The listing builds one solid part. Answer for the finished solid, in the listing's coordinates (mm). A direction names the side the tool comes from. Give positions to 0.01 mm unless a question says otherwise; leave off trailing zeros. Write each loop counter-clockwise with the first axis right and the second up, starting at its lowest first coordinate (ties: lowest second). Pieces come first, ordered by that corner, then holes. Notation, with made-up numbers: (78, 78) -> (131, 78) arc R13 ccw to (131, 82) -> close; hole circle Ø11 at (62, 85). An arc over 180 degrees is marked (long way). Use CSV: the item, a comma, the result in double quotes. Start each with the question number.
from build123d import *

# Parameters (mm, degrees)
BOSS_EXTRUDE1_DEPTH     = 6.35
CUT_EXTRUDE1_START      = -9.525
SKETCH2_R               = 2.286
SKETCH2_R_2             = 2.285999999999999
CUT_EXTRUDE1_DEPTH      = 19.05
CUT_EXTRUDE2_DEPTH      = 15.892070207999966
CUT_EXTRUDE2_DEPTH_BACK = 15.892070207999966
SKETCH3_R               = 2.286
BOSS_EXTRUDE2_DEPTH     = 3.048
BOSS_EXTRUDE3_REACH     = 17.642
FILLET1_R               = 2.54
FILLET2_R               = 0.762


with BuildPart() as part:
    # Sketch1 → Boss-Extrude1 (new body)
    with BuildSketch(Plane(origin=(0, 0, 0), x_dir=(1, 0, 0), z_dir=(0, 1, 0))):
        with BuildLine():
            Line((6.984999999999984, -9.525000000000002), (-6.98499999999998, -9.525000000000006))
            ThreePointArc((-6.98499999999998, -9.525000000000006), (-8.78105122421383, -8.781051224213837), (-9.524999999999999, -6.984999999999987))
            Line((-9.524999999999999, -6.984999999999987), (-9.524999999999999, 6.984999999999979))
            ThreePointArc((-9.524999999999999, 6.984999999999979), (-8.78105122421383, 8.781051224213828), (-6.984999999999981, 9.524999999999997))
            Line((-6.984999999999981, 9.524999999999997), (6.984999999999984, 9.525))
            ThreePointArc((6.984999999999984, 9.525), (8.781051224213833, 8.781051224213831), (9.525000000000002, 6.984999999999983))
            Line((9.525000000000002, 6.984999999999983), (9.525000000000002, -6.984999999999984))
            ThreePointArc((9.525000000000002, -6.984999999999984), (8.781051224213833, -8.781051224213833), (6.984999999999984, -9.525000000000002))
        make_face()
    extrude(amount=BOSS_EXTRUDE1_DEPTH)

    # Sketch2 → Cut-Extrude1 (cut)
    with BuildSketch(Plane.XY.offset(CUT_EXTRUDE1_START)):
        with Locations(Location((-4.7624999999999975, 3.175, 0), (0, 0, 166.463797263))):
            Circle(SKETCH2_R)
        with Locations(Location((4.762500000000003, 3.175, 0), (0, 0, 13.536202737))):
            Circle(SKETCH2_R_2)
    extrude(amount=CUT_EXTRUDE1_DEPTH, mode=Mode.SUBTRACT)

    # Sketch3 → Cut-Extrude2 (cut, two sides: drawn at the far end of the back side and taken through both)
    with BuildSketch(Plane(origin=(0, 0, 0), x_dir=(0, 0, -1), z_dir=(1, 0, 0)).offset(-CUT_EXTRUDE2_DEPTH_BACK)):
        with Locations(Location((-4.7625, 3.175, 0), (0, 0, 90))):
            Circle(SKETCH3_R)
        with Locations(Location((4.7625, 3.175, 0), (0, 0, 90))):
            Circle(SKETCH3_R)
    extrude(amount=CUT_EXTRUDE2_DEPTH + CUT_EXTRUDE2_DEPTH_BACK, mode=Mode.SUBTRACT)


with BuildPart() as body_2:
    # Sketch4 → Boss-Extrude2 (new, symmetric)
    with BuildSketch(Plane.XY):
        Polygon((-6.35, -3.175), (6.35, -3.1749999999999985), (6.350000000000001, -4.775199999999996), (3.175, -7.950199999999998), (-3.174999999999998, -7.950199999999998), (-6.35, -4.775199999999998), align=None)
    extrude(amount=BOSS_EXTRUDE2_DEPTH, both=True)

    # Sketch5 → Boss-Extrude3 (add, up to next)
    with BuildSketch(Plane.XZ, mode=Mode.PRIVATE) as boss_extrude3_sk1:
        with BuildLine():
            Line((3.0479999999999996, -3.0479999999999996), (0, -3.048))
            ThreePointArc((0, -3.048), (-2.155261469056597, -2.155261469056597), (-3.0479999999999996, 4.3e-16))
            Line((-3.0479999999999996, 4.3e-16), (-3.048000000000001, 3.048))
            Line((-3.048000000000001, 3.048), (0, 3.048))
            ThreePointArc((0, 3.048), (2.1552614690565965, 2.155261469056597), (3.0479999999999996, 4.3e-16))
            Line((3.0479999999999996, 4.3e-16), (3.0479999999999996, -3.0479999999999996))
        make_face()
    boss_extrude3_tool1 = extrude(boss_extrude3_sk1.sketch, amount=BOSS_EXTRUDE3_REACH, mode=Mode.PRIVATE) - body_2.part

    add(part.part)  # Boss-Extrude3 merges part
    add(boss_extrude3_tool1.solids().sort_by_distance((0, 0, 0))[0])

    # Sketch6 → Revolve1 (revolve)
    with BuildSketch(Plane.XY):
        with BuildLine():
            Line((-6.349999999999999, -1.016), (-6.349999999999999, 0))
            Line((-6.349999999999999, 0), (-8.889999999999999, 0))
            ThreePointArc((-8.889999999999999, 0), (-7.717831861012163, -0.7525796525304105), (-6.349999999999999, -1.016))
        make_face()
    revolve1 = revolve(axis=Axis((-6.349999999999999, 0, 0), (0, 1, 0)))

    # Mirror1: Revolve1 across plane
    add(revolve1.mirror(Plane(origin=(0, 0, 0), x_dir=(0, 0, 1), z_dir=(1, 0, 0))))

    # Fillet1
    fillet1_edges = [body_2.edges().sort_by_distance(p)[0] for p in [
        (-6.35, -3.975099999999999, -3.048),
        (6.3500000000000005, -3.9750999999999976, 3.048),
    ]]
    fillet(fillet1_edges, radius=FILLET1_R)

    # Fillet2
    # the kernel refuses this fillet: 0.762 mm, written as the material it adds along each edge
    with BuildSketch(Plane(origin=(-6.349999999999999, 0, 0), x_dir=(-1, 0, 0), z_dir=(0, 0, -1))) as fillet2_piece_1:
        with BuildLine():
            CenterArc((2.8284242963176522, -0.762), FILLET2_R, 90, 39.51765279717284)
            ThreePointArc((2.3435515598060546, -0.17417142857142887), (2.443328238479981, -0.08883673664575209), (2.54, 0))
            Line((2.54, 0), (2.8284242963176522, 0))
        make_face()
    revolve(axis=Axis((-6.349999999999999, 0, 0), (0, 1, 0)))
    with BuildSketch(Plane(origin=(6.349999999999999, 0, 0), x_dir=(1, 0, 0), z_dir=(0, 0, -1))) as fillet2_piece_2:
        with BuildLine():
            CenterArc((2.8284242963176522, 0.762), FILLET2_R, 230.48234720282716, 39.51765279717284)
            ThreePointArc((2.3435515598060546, 0.17417142857142887), (2.443328238479981, 0.08883673664575209), (2.54, 0))
            Line((2.54, 0), (2.8284242963176522, 0))
        make_face()
    revolve(axis=Axis((6.349999999999999, 0, 0), (0, -1, 0)))
    # the kernel refuses this fillet: 0.762 mm, written as the material it takes off along each edge
    with BuildSketch(Plane(origin=(3.0479999999999996, 0, -3.0479999999999996), x_dir=(0, 0, 1), z_dir=(0, -1, 0))) as fillet2_2_piece_1:
        with BuildLine():
            CenterArc((FILLET2_R, FILLET2_R), FILLET2_R, 180, 90)
            Line((0, FILLET2_R), (0, 0))
            Line((0, 0), (FILLET2_R, 0))
        make_face()
    extrude(amount=3.174999999999999, mode=Mode.SUBTRACT)
    with BuildSketch(Plane(origin=(-3.048000000000001, 0, 3.048), x_dir=(1, 0, 0), z_dir=(0, -1, 0))) as fillet2_2_piece_2:
        with BuildLine():
            CenterArc((FILLET2_R, -FILLET2_R), FILLET2_R, 90, 90)
            Line((4.4e-16, -FILLET2_R), (0, 0))
            Line((0, 0), (FILLET2_R, 0))
        make_face()
    extrude(amount=3.1749999999999994, mode=Mode.SUBTRACT)
    # the kernel refuses this fillet: 0.762 mm, written as the material it adds along each edge
    with BuildSketch(Plane(origin=(-7.8e-16, 0, -1.55e-15), x_dir=(2.5e-16, 0, -1), z_dir=(1, 0, 2.5e-16))) as fillet2_3_piece_1:
        with BuildLine():
            CenterArc((3.0479999999999983 + FILLET2_R, -FILLET2_R), FILLET2_R, 90, 90)
            Line((3.0479999999999983 + FILLET2_R, 1.1e-16), (3.0479999999999983, 0))
            Line((3.0479999999999983, 0), (3.0479999999999983, -FILLET2_R))
        make_face()
    revolve(axis=Axis((-7.8e-16, 0, -1.55e-15), (0, 1, 0)), revolution_arc=90.00000000000006)
    with BuildSketch(Plane(origin=(2.2859999999999996, 0, -3.0479999999999996), x_dir=(0, -1, -5.8e-16), z_dir=(-1, 0, -1.5e-16))) as fillet2_3_piece_2:
        with BuildLine():
            CenterArc((FILLET2_R, -FILLET2_R), FILLET2_R, 90.00000000000004, 89.99999999999996)
            Line((0, -FILLET2_R), (0, 0))
            Line((0, 0), (FILLET2_R, 0))
        make_face()
    extrude(amount=2.2859999999999996)
    with BuildSketch(Plane(origin=(3.0479999999999996, 0, 4.3e-16), x_dir=(0, -1, 0), z_dir=(0, 0, -1))) as fillet2_3_piece_3:
        with BuildLine():
            CenterArc((FILLET2_R, -FILLET2_R), FILLET2_R, 90, 90)
            Line((-1.1e-16, -FILLET2_R), (0, 0))
            Line((0, 0), (FILLET2_R, 0))
        make_face()
    extrude(amount=2.286)
    with BuildSketch(Plane(origin=(-3.0479999999999996, 0, 4.3e-16), x_dir=(0, -1, 0), z_dir=(-4.4e-16, 0, 1))) as fillet2_3_piece_4:
        with BuildLine():
            CenterArc((FILLET2_R, -FILLET2_R), FILLET2_R, 90, 90)
            Line((-1.1e-16, -FILLET2_R), (0, 0))
            Line((0, 0), (FILLET2_R, 0))
        make_face()
    extrude(amount=2.285999999999999)
    with BuildSketch(Plane(origin=(-2.2e-16, 0, 2.2e-16), x_dir=(7e-17, 0, 1), z_dir=(-1, 0, 7e-17))) as fillet2_3_piece_5:
        with BuildLine():
            CenterArc((3.048 + FILLET2_R, -FILLET2_R), FILLET2_R, 90, 90)
            Line((3.048 + FILLET2_R, 1.1e-16), (3.048, 0))
            Line((3.048, 0), (3.048, -FILLET2_R))
        make_face()
    revolve(axis=Axis((-2.2e-16, 0, 2.2e-16), (0, 1, 0)), revolution_arc=90)
    with BuildSketch(Plane(origin=(-2.2860000000000005, 0, 3.048), x_dir=(0, -1, 0), z_dir=(1, 0, 0))) as fillet2_3_piece_6:
        with BuildLine():
            CenterArc((FILLET2_R, -FILLET2_R), FILLET2_R, 90, 90)
            Line((-4.4e-16, -FILLET2_R), (0, 0))
            Line((0, 0), (FILLET2_R, 0))
        make_face()
    extrude(amount=2.2860000000000005)
    with BuildSketch(Plane(origin=(-2.2860000000000005, 0, 2.286), x_dir=(0, 0, 1), z_dir=(1, 0, 0))) as fillet2_3_piece_7:
        with BuildLine():
            CenterArc((0.762 + FILLET2_R, FILLET2_R), FILLET2_R, 180, 90)
            Line((0.762, FILLET2_R), (0.762, 0))
            Line((0.762, 0), (0.762 + FILLET2_R, 0))
        make_face()
    revolve(axis=Axis((-2.2860000000000005, 0, 2.286), (0, -1, 0)), revolution_arc=90.00000000000004)
    with BuildSketch(Plane(origin=(2.2859999999999996, 0, -2.2859999999999996), x_dir=(1, 0, 0), z_dir=(0, 0, 1))) as fillet2_3_piece_8:
        with BuildLine():
            CenterArc((0.762 + FILLET2_R, -FILLET2_R), FILLET2_R, 90, 90)
            Line((0.762 + FILLET2_R, 1.1e-16), (0.762, 0))
            Line((0.762, 0), (0.762, -FILLET2_R))
        make_face()
    revolve(axis=Axis((2.2859999999999996, 0, -2.2859999999999996), (0, 1, 0)), revolution_arc=90)


solid = body_2.part
Q1. For faces 5 (the face through (-7.71, 1.49, -3.22)), 6 (the face through (-1, -5, 3.048)), 7 (the face through (-3.486, 1.279, 7.64)), 8 (the face through (6.35, -4, -1)), 9 (the face through (1, -5, -3.048)), determine the directions among +Z, -Z, +X, -X, +Y, -Y from which every point of the face is accessible in a straight line to the end or side of a thin tool.
Q2. The mould has two halves that part along Z. Classify faces 1 (the face through (5, -3.175, 0)), 2 (the face through (7.64, 1.49, 6.31)), 3 (the face through (8.76, 3.13, -8.8)), 4 (the face through (-0.07, 0.89, 4.86)): +Z half, -Z half, draft (parallel to the pull), parting line (faces both ways), or undercut.
Q3. Straight lines are drawn through the part: L1, parallel to X at y = 5.25, z = -7; L2, parallel to Z at x = 8, y = 4.75; L3, parallel to X at y = 4, z = 1 (3 decimals). For each, find the intervals that lie inside material, in ascending order.
Q4. Section B-B on y = -4 is taken. Give the vertices of the cut face in (x, z), then the cut area to 4 significant figures.
Q5. Flat-ended cylindrical pins translate along their axes: pin 1 Ø1.1 at (y, z) = (-2, 1.5) entering from -X; pin 2 Ø6 at (x, z) = (-6.5, -4) entering from -Y; pin 3 Ø0.8 at (y, z) = (-4, 1.5) entering from -X. Find the tip coordinate at first contact, or state that the pin passes through.
Q6. Section A-A on z = -8 is taken. State how many separate pieces and enclosed holes the cut face has, then the cut area to 3 significant figures.
Output:
1,face 5,"+X, -X"
1,face 6,"+Z, +X, -X, -Y"
1,face 7,"+Z, -Z"
1,face 8,"+Z, -Z, +X, -Y"
1,face 9,"-Z, +X, -X, -Y"
2,face 1,"draft"
2,face 2,"undercut"
2,face 3,"-Z half"
2,face 4,"undercut"
3,L1,"-9.52 to -5.72, -3.8 to 3.8, 5.72 to 9.52"
3,L2,"-9.31 to -6.42, -3.11 to 3.11, 6.42 to 9.31"
3,L3,"-9.525 to -6.894, -2.631 to 2.631, 6.894 to 9.525"
4,outline,"(-6.35, -0.51) arc R2.54 ccw to (-3.81, -3.05) -> (6.35, -3.05) -> (6.35, 0.51) arc R2.54 ccw to (3.81, 3.05) -> (-6.35, 3.05) -> close"
4,area,"74.65 mm²"
5,pin 1,"x = -3.05"
5,pin 2,"y = -7.47"
5,pin 3,"x = -6.35"
6,separate pieces,"1"
6,enclosed holes,"2"
6,area,"85.4 mm²"
